Model file for the job. Use its own axes, mm. A direction names the side the tool comes from. Coordinates: 2 decimals unless noted, no trailing zeros. Return JSON: item names as keys, results as strings.
```python
from build123d import *

# Parameters (mm, degrees)
SKETCH2_R           = 3.175
BOSS_EXTRUDE1_DEPTH = 6.35


with BuildPart() as part:
    # Sketch2 → Boss-Extrude1 (new body)
    with BuildSketch(Plane.XY):
        with BuildLine():
            add(Edge.make_bspline(
                [(88.748610912, 21.468378691), (87.390018144, 29.081992428), (95.098610912, 30.993378691)],
                knots=[0, 0, 0, 1, 1, 1], degree=2))
            Line((95.098610912, 30.993378691), (95.098610912, 27.818378691))
            ThreePointArc((95.098610912, 27.818378691), (99.588738973, 25.958506751), (101.448610912, 21.468378691))
            add(Edge.make_bspline(
                [(101.448610912, 21.468378691), (102.807203681, 13.854764953), (95.098610912, 11.943378691)],
                knots=[0, 0, 0, 1, 1, 1], degree=2))
            Line((95.098610912, 11.943378691), (95.098610912, 15.118378691))
            ThreePointArc((95.098610912, 15.118378691), (90.608482852, 16.97825063), (88.748610912, 21.468378691))
        make_face()
        with Locations((95.098610912, 21.468378691)):
            Circle(SKETCH2_R, mode=Mode.SUBTRACT)
    extrude(amount=BOSS_EXTRUDE1_DEPTH)


solid = part.part
```
Item 1: Pull direction X, two halves, no side cores. Call faces 1 (the flat face through (95.099, 14, 3)), 2 (the cylindrical face through (99.539, 26.008, 3.131)), 3 (the flat face through (99, 22, 6.35)), 4 (the cylindrical face through (92.579, 19.536, 3.131)): +X half, -X half, draft (parallel to the pull), parting line (faces both ways), or undercut.
Check result:
{"face 1": "-X half", "face 2": "+X half", "face 3": "draft", "face 4": "undercut"}
Item 2: 3-axis set-ups, long thin cutter, end or side, ignore diameter. For faces 5 (the cylindrical face through (90.66, 16.93, 3.13)), 6 (the flat face through (95.099, 29, 3)): which of +Z, -Z, +X, -X, +Y, -Y reach the whole face in a straight line?
Check result:
{"face 5": "+Z, -Z, -X, -Y", "face 6": "+Z, -Z, +X, +Y"}
Item 3: Drop flat-ended pins along their axis: pin 1 Ø3 at (x, z) = (100, 5.5) entering from +Y; pin 2 Ø1 at (y, z) = (14, 2.5) entering from -X. Give the stop position or say it passes through.
Check result:
{"pin 1": "stops at y = 26.83", "pin 2": "stops at x = 95.1"}
Item 4: Wall check: line 1 (X direction, y = 21.5, z = 4.75); line 2 (Y direction, x = 97, z = 0.5); line 3 (X direction, y = 22.5, z = 4). Give the ranges that are in metal, low to high.
Check result:
{"line 1": "x = 88.74 to 91.92, 98.27 to 101.45", "line 2": "y = 12.56 to 18.93, 24.01 to 27.53", "line 3": "x = 88.6 to 92.1, 98.1 to 101.36"}
